Part print with two shaded views. Sizes in mm from the minimum x, y, z corner. Coordinates: 2 decimals unless noted, no trailing zeros. Loops run counter-clockwise (first coordinate to the right, second up) from the corner with the lowest first, then second, coordinate; pieces in that order, holes last. Notation, with made-up numbers: (51, 7) -> (97, 7) arc R27 cw to (97, 41) -> close; hole circle Ø10 at (82, -4.5). An arc over 180 degrees is marked (long way). One line per item, written item: value. Start each with the question number.
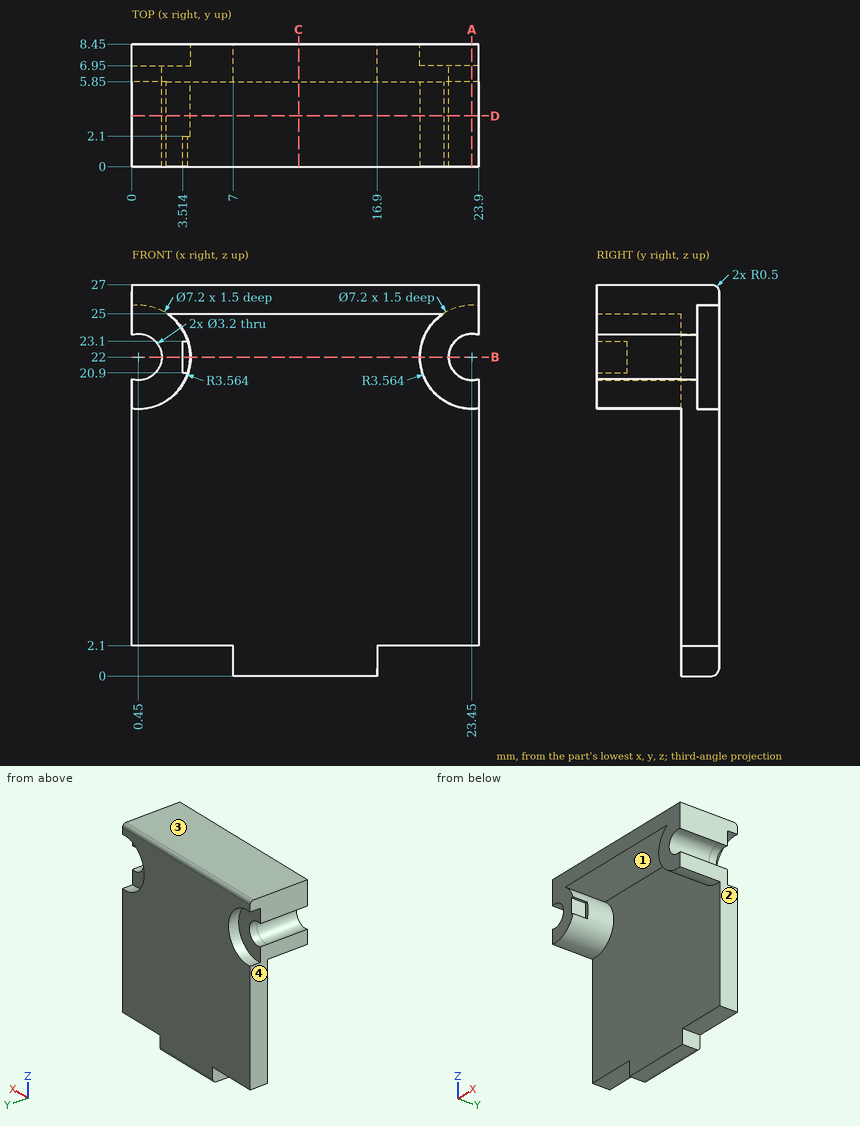
Item 1: Two-plate mould, pull along X, no slides. Class the marked faces 1, 2, 3 and 4: +X half, -X half, draft (parallel to the pull), parting line (faces both ways), or undercut.
Item 2: Band-saw the part on D-D, the plane y = 3.5. List the corners of the cut face in (x, z).
Item 3: Probe probe 1 along Z at (x, y) = (23.45, 6.35); probe 2 along Z at (x, y) = (0.45, 2.5); probe 3 along Y at (x, z) = (14.25, 15.75). List the from-to ranges inside material, lowest first.
Item 4: Band-saw the part on A-A, the plane x = 23.45. List the corners of the cut face in (y, z).
Item 5: Band-saw the part on B-B, the plane z = 22. List the corners of the cut face in (x, y).
Item 6: Band-saw the part on C-C, the plane x = 11.5. List the corners of the cut face in (y, z), and give its area (3 significant figures).
Item 7: Drop flat-ended pins along their axis: pin 1 Ø2 at (x, y) = (21, 7.5) entering from -Z; pin 2 Ø1 at (x, y) = (21, 1) entering from -Z; pin 3 Ø1.2 at (x, z) = (22, 22.5) entering from +Y. Give the stop position or say it passes through.
Worked out:
1. face 1: undercut
1. face 2: +X half
1. face 3: draft
1. face 4: -X half
2. outline: (0, 18.46) arc R3.56 ccw to (2.37, 25) -> (21.53, 25) arc R3.56 ccw to (23.9, 18.46) -> (23.9, 20.46) arc R1.6 cw (long way) to (23.9, 23.54) -> (23.9, 27) -> (0, 27) -> (0, 23.54) arc R1.6 cw (long way) to (0, 20.46) -> close
3. probe 1: z = 2.1 to 20.4, 23.6 to 27
3. probe 2: z = 18.44 to 20.4, 23.6 to 27
3. probe 3: y = 5.85 to 8.45
4. outline: (0, 18.44) -> (5.85, 18.44) -> (5.85, 2.1) -> (8.45, 2.1) -> (8.45, 18.4) -> (6.95, 18.4) -> (6.95, 20.4) -> (0, 20.4) -> close; (0, 23.6) -> (6.95, 23.6) -> (6.95, 25.6) -> (8.45, 25.6) -> (8.45, 26.5) arc R0.5 ccw to (7.95, 27) -> (0, 27) -> close
5. outline: (2.05, 0) -> (3.51, 0) -> (3.51, 2.1) -> (4.01, 2.1) -> (4.01, 5.85) -> (19.89, 5.85) -> (19.89, 0) -> (21.85, 0) -> (21.85, 6.95) -> (19.85, 6.95) -> (19.85, 8.45) -> (4.05, 8.45) -> (4.05, 6.95) -> (2.05, 6.95) -> close
6. outline: (0, 25) -> (5.85, 25) -> (5.85, 0) -> (7.95, 0) arc R0.5 ccw to (8.45, 0.5) -> (8.45, 26.5) arc R0.5 ccw to (7.95, 27) -> (0, 27) -> close
6. area: 81.8 mm²
7. pin 1: stops at z = 2.1
7. pin 2: stops at z = 19.02
7. pin 3: stops at y = 6.95
